Verification items for the finished model (mm, model axes). A direction names the side the tool comes from. Give positions to 0.01 mm unless a question says otherwise; leave off trailing zeros. Write each loop counter-clockwise with the first axis right and the second up, starting at its lowest first coordinate (ties: lowest second). Pieces come first, ordered by that corner, then holes.
from build123d import *

# Parameters (mm, degrees)
SKETCH_1_R          = 18
EXTRUDE_1_DEPTH     = 3
SKETCH_2_R          = 1.5
CUT_EXTRUDE_1_DEPTH = 3
SKETCH_4_W          = 15
SKETCH_4_H          = 3
EXTRUDE_2_DEPTH     = 8
SKETCH_5_R          = 1.5
CUT_EXTRUDE_2_DEPTH = 37
FILLET_1_R          = 3
FILLET_2_R          = 1
SKETCH_6_R          = 6
CUT_EXTRUDE_3_DEPTH = 37


with BuildPart() as part:
    # Эскиз1 → Бобышка-Вытянуть1 (new body)
    with BuildSketch(Plane.XY):
        Circle(SKETCH_1_R)
    extrude(amount=EXTRUDE_1_DEPTH)

    # Эскиз2 → Вырез-Вытянуть1 (cut)
    with BuildSketch(Plane.XY.offset(3)):
        with Locations((-10.606601718, -10.606601718)):
            Circle(SKETCH_2_R)
        with Locations((10.606601718, -10.606601718)):
            Circle(SKETCH_2_R)
        with Locations((10.606601718, 10.606601718)):
            Circle(SKETCH_2_R)
        with Locations((-10.606601718, 10.606601718)):
            Circle(SKETCH_2_R)
    extrude(amount=-CUT_EXTRUDE_1_DEPTH, mode=Mode.SUBTRACT)

    # Эскиз4 → Бобышка-Вытянуть2 (add)
    with BuildSketch(Plane.XY.offset(3)):
        with Locations((0, 14.863068172)):
            Rectangle(SKETCH_4_W, SKETCH_4_H)
        with Locations((0, -14.863068172)):
            Rectangle(SKETCH_4_W, SKETCH_4_H)
    extrude(amount=EXTRUDE_2_DEPTH)

    # Эскиз5 → Вырез-Вытянуть2 (cut)
    with BuildSketch(Plane(origin=(0, 16.363068172, 0), x_dir=(1, 0, 0), z_dir=(0, 1, 0))):
        with Locations(Location((-4.5, -7, 0), (0, 0, 270))):
            Circle(SKETCH_5_R)
        with Locations(Location((4.5, -7, 0), (0, 0, 270))):
            Circle(SKETCH_5_R)
    extrude(amount=-CUT_EXTRUDE_2_DEPTH, mode=Mode.SUBTRACT)

    # Скругление1
    fillet_1_edges = [part.edges().sort_by_distance(p)[0] for p in [
        (-7.5, 14.863068172, 11),
        (7.5, 14.863068172, 11),
        (7.5, -14.863068172, 11),
        (-7.5, -14.863068172, 11),
    ]]
    fillet(fillet_1_edges, radius=FILLET_1_R)

    # Скругление2
    # the kernel refuses this fillet: 1 mm, written as the material it adds along each edge
    with BuildSketch(Plane(origin=(-7.5, 16.363068172, 3), x_dir=(-1, 0, 0), z_dir=(0, -1, 0))) as fillet_2_piece_1_section:
        with BuildLine():
            CenterArc((FILLET_2_R, -FILLET_2_R), FILLET_2_R, 90, 90)
            Line((0, -FILLET_2_R), (0, 0))
            Line((0, 0), (FILLET_2_R, 0))
        make_face()
    fillet_2_piece_1 = extrude(amount=3, mode=Mode.PRIVATE)
    fillet_2_piece_1 = fillet_2_piece_1 & Plane(origin=(0, 0, 3.230923565), x_dir=(1, 0, 0), z_dir=(0, 0, -1)) * Cylinder(18, 11, mode=Mode.PRIVATE)
    add(fillet_2_piece_1)
    with BuildSketch(Plane(origin=(7.5, 13.363068172, 3), x_dir=(1, 0, 0), z_dir=(0, 1, 0))) as fillet_2_piece_2_section:
        with BuildLine():
            CenterArc((FILLET_2_R, -FILLET_2_R), FILLET_2_R, 90, 90)
            Line((0, -FILLET_2_R), (0, 0))
            Line((0, 0), (FILLET_2_R, 0))
        make_face()
    fillet_2_piece_2 = extrude(amount=3, mode=Mode.PRIVATE)
    fillet_2_piece_2 = fillet_2_piece_2 & Plane(origin=(0, 0, 3.230923565), x_dir=(1, 0, 0), z_dir=(0, 0, -1)) * Cylinder(18, 10, mode=Mode.PRIVATE)
    add(fillet_2_piece_2)
    with BuildSketch(Plane(origin=(7.5, -16.363068172, 3), x_dir=(0, 0, 1), z_dir=(0, 1, 0))) as fillet_2_piece_3_section:
        with BuildLine():
            CenterArc((FILLET_2_R, FILLET_2_R), FILLET_2_R, 180, 90)
            Line((0, FILLET_2_R), (0, 0))
            Line((0, 0), (FILLET_2_R, 0))
        make_face()
    fillet_2_piece_3 = extrude(amount=3, mode=Mode.PRIVATE)
    fillet_2_piece_3 = fillet_2_piece_3 & Plane(origin=(0, 0, 3.230923542), x_dir=(1, 0, 0), z_dir=(0, 0, -1)) * Cylinder(18, 10, mode=Mode.PRIVATE)
    add(fillet_2_piece_3)
    with BuildSketch(Plane(origin=(-7.5, -13.363068172, 3), x_dir=(-1, 0, 0), z_dir=(0, -1, 0))) as fillet_2_piece_4_section:
        with BuildLine():
            CenterArc((FILLET_2_R, -FILLET_2_R), FILLET_2_R, 90, 90)
            Line((0, -FILLET_2_R), (0, 0))
            Line((0, 0), (FILLET_2_R, 0))
        make_face()
    fillet_2_piece_4 = extrude(amount=3, mode=Mode.PRIVATE)
    fillet_2_piece_4 = fillet_2_piece_4 & Plane(origin=(0, 0, 3.230923565), x_dir=(1, 0, 0), z_dir=(0, 0, -1)) * Cylinder(18, 11, mode=Mode.PRIVATE)
    add(fillet_2_piece_4)

    # Эскиз6 → Вырез-Вытянуть3 (cut)
    with BuildSketch(Plane.XY.offset(3)):
        Circle(SKETCH_6_R)
    extrude(amount=-CUT_EXTRUDE_3_DEPTH, mode=Mode.SUBTRACT)


solid = part.part
Item 1: Set-up check for faces 4 (the face through (0, -13.363, 7)), 5 (the face through (7.5, 15, 6)), 6 (the face through (0, 17, 3)), 7 (the face through (-7.5, 15, 6)): record each of +Z, -Z, +X, -X, +Y, -Y from which the full face is reachable in a straight line by a thin tool's end or side.
Answer key:
face 4: +Z, +X, -X
face 5: +Z, +X, +Y, -Y
face 6: +Z, +X, -X, +Y
face 7: +Z, -X, +Y, -Y
Item 2: Sectioned sample at A-A on x = 0. Record the cut outline in (y, z), then the cut area to 3 significant figures.
Answer key:
outline: (-18, 0) - (-6, 0) - (-6, 3) - (-13.36, 3) - (-13.36, 11) - (-16.36, 11) - (-16.36, 3) - (-18, 3) - close; (6, 0) - (18, 0) - (18, 3) - (16.36, 3) - (16.36, 11) - (13.36, 11) - (13.36, 3) - (6, 3) - close
area: 120 mm2
Item 3: Sectioned sample at C-C on y = 0. Record the cut outline in (x, z), then the cut area to 3 significant figures.
Answer key:
outline: (-18, 0) - (-6, 0) - (-6, 3) - (-18, 3) - close; (6, 0) - (18, 0) - (18, 3) - (6, 3) - close
area: 72.0 mm2
Item 4: Depth check by flat-ended pin: pin 1 (0.8 mm diameter, centred on x = 2, y = -17.5, fed in from +Z); pin 2 (0.9 mm diameter, centred on y = 14, z = 6, fed in from -X); pin 3 (4 mm diameter, centred on y = 12, z = 3.5, fed in from +X); pin 4 (3 mm diameter, centred on y = 2.5, z = 5, fed in from +X). Enter the tip coordinate at first touch or a pass-through.
Answer key:
pin 1: stops at z = 3
pin 2: stops at x = -7.5
pin 3: stops at x = 14.92
pin 4: passes through
Item 5: Release check for a two-part mould opening along X. For faces 1 (the face through (-4.43, -14.84, 5.5)), 2 (the face through (-7.801, -14.842, 3.285)), 3 (the face through (0, -7, 3)) record: released by +X, released by -X, zero draft, split by the parting line, or undercut.
Answer key:
face 1: undercut
face 2: released by -X
face 3: zero draft
Item 6: Scan lines: line 1 along X through (y, z) = (-14.2, 7); line 2 along Y through (x, z) = (0, 9); line 3 along Y through (x, z) = (0, 0.9). Record each from-to range of solid material in increasing order.
Answer key:
line 1: x = -7.5 to -6, -3 to 3, 6 to 7.5
line 2: y = -16.36 to -13.36, 13.36 to 16.36
line 3: y = -18 to -6, 6 to 18
Item 7: Sectioned sample at D-D on z = 7. Record the cut outline in (x, y).
Answer key:
outline: (-7.5, -16.36) - (-6, -16.36) - (-6, -13.36) - (-7.5, -13.36) - close; (-7.5, 13.36) - (-6, 13.36) - (-6, 16.36) - (-7.5, 16.36) - close; (-3, -16.36) - (3, -16.36) - (3, -13.36) - (-3, -13.36) - close; (-3, 13.36) - (3, 13.36) - (3, 16.36) - (-3, 16.36) - close; (6, -16.36) - (7.5, -16.36) - (7.5, -13.36) - (6, -13.36) - close; (6, 13.36) - (7.5, 13.36) - (7.5, 16.36) - (6, 16.36) - close
Item 8: Sectioned sample at B-B on z = 4.5. Record the cut outline in (x, y), then the cut area to 3 significant figures.
Answer key:
outline: (-7.5, -16.36) - (7.5, -16.36) - (7.5, -13.36) - (-7.5, -13.36) - close; (-7.5, 13.36) - (7.5, 13.36) - (7.5, 16.36) - (-7.5, 16.36) - close
area: 90.0 mm2
